from build123d import *

# Parameters (mm, degrees)
SKIZZE1_R                       = 48.5
AUFSATZ_LINEAR_AUSTRAGEN1_DEPTH = 5
SKIZZE2_W                       = 20
SKIZZE2_H                       = 13
AUFSATZ_LINEAR_AUSTRAGEN2_DEPTH = 20
SKIZZE3_W                       = 20
SKIZZE3_H                       = 2
AUFSATZ_LINEAR_AUSTRAGEN3_DEPTH = 23
SKIZZE4_R                       = 2.1
SCHNITT_LINEAR_AUSTRAGEN1_DEPTH = 74.003424577
FASE4_SIZE                      = 0.6
FASE6_SIZE                      = 2.5


with BuildPart() as part:
    # Skizze1 → Aufsatz-Linear austragen1 (new body)
    with BuildSketch(Plane(origin=(0, 0, 0), x_dir=(1, 0, 0), z_dir=(0, 1, 0))):
        with Locations(Location((0, 0, 0), (0, 0, 270))):
            Circle(SKIZZE1_R)
    extrude(amount=AUFSATZ_LINEAR_AUSTRAGEN1_DEPTH)

    # Skizze2 → Aufsatz-Linear austragen2 (add)
    with BuildSketch(Plane.XZ):
        with Locations((-27.5, 0)):
            Rectangle(SKIZZE2_W, SKIZZE2_H)
    extrude(amount=AUFSATZ_LINEAR_AUSTRAGEN2_DEPTH)

    # Skizze3 → Aufsatz-Linear austragen3 (add)
    with BuildSketch(Plane.XZ):
        with Locations((-27.5, 7.5)):
            Rectangle(SKIZZE3_W, SKIZZE3_H)
        with Locations((-27.5, -7.5)):
            Rectangle(SKIZZE3_W, SKIZZE3_H)
    extrude(amount=AUFSATZ_LINEAR_AUSTRAGEN3_DEPTH)

    # Skizze4 → Schnitt-Linear austragen1 (cut, through all)
    with BuildSketch(Plane.XZ.offset(20)):
        with Locations(Location((-32.5, 0, 0), (0, 0, 270))):
            Circle(SKIZZE4_R)
        with Locations(Location((-22.5, 0, 0), (0, 0, 270))):
            Circle(SKIZZE4_R)
    extrude(amount=-SCHNITT_LINEAR_AUSTRAGEN1_DEPTH, mode=Mode.SUBTRACT)

    # Fase4
    fase4_edges = [part.edges().sort_by_distance(p)[0] for p in [
        (0, 5, -48.5),
    ]]
    chamfer(fase4_edges, length=FASE4_SIZE)

    # Fase6
    fase6_edges = [part.edges().sort_by_distance(p)[0] for p in [
        (-32.5, 5, 2.1),
        (-22.5, 5, 2.1),
    ]]
    chamfer(fase6_edges, length=FASE6_SIZE)


solid = part.part
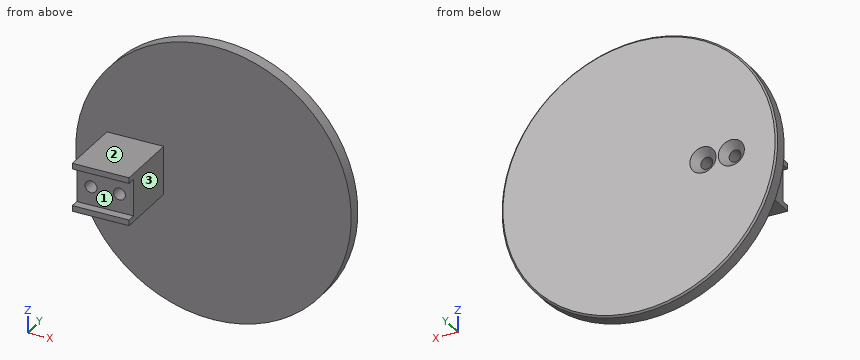
Geometry check sheet. Reference: the model listing, model coordinates, mm. Face numbers are marked on the shaded views. Give positions to 0.01 mm unless a question says otherwise; leave off trailing zeros. Write each loop counter-clockwise with the first axis right and the second up, starting at its lowest first coordinate (ties: lowest second). Pieces come first, ordered by that corner, then holes. Notation, with made-up numbers: M 81,86 L 97,86 A20 ccw 97,124 Z; hole C 22,55.5 d7. An arc over 180 degrees is marked long. One line per question, with ' | ' between items.
1. Cross-section at C-C (x = 0). Enter the section's corners in (y, z).
Ans:
outline: M 0,-48.5 L 4.4,-48.5 L 5,-47.9 L 5,47.9 L 4.4,48.5 L 0,48.5 Z
2. Cross-section at B-B (y = -12.75). Enter the section's corners in (x, z).
Ans:
outline: M -37.5,-8.5 L -17.5,-8.5 L -17.5,8.5 L -37.5,8.5 Z; hole C -32.5,0 d4.2; hole C -22.5,0 d4.2
3. Scan lines: line 1 along X through (y, z) = (-14.5, 0); line 2 along Y through (x, z) = (-24, -13); line 3 along X through (y, z) = (-1.5, 5.5). Record each from-to range of solid material in increasing order. Write a range as from..to.
Ans:
line 1: -37.5..-34.6, -30.4..-24.6, -20.4..-17.5 | line 2: 0..5 | line 3: -37.5..-17.5
4. Cross-section at A-A (z = 0). Enter the section's corners in (x, y).
Ans:
outline: M -48.5,0 L -37.5,0 L -37.5,-20 L -34.6,-20 L -34.6,2.5 L -37.1,5 L -47.9,5 L -48.5,4.4 Z; M -30.4,-20 L -24.6,-20 L -24.6,2.5 L -27.1,5 L -27.9,5 L -30.4,2.5 Z; M -20.4,-20 L -17.5,-20 L -17.5,0 L 48.5,0 L 48.5,4.4 L 47.9,5 L -17.9,5 L -20.4,2.5 Z
5. Mould release check, pull along Z, two halves, no side actions. Record for the marked faces 1, 2 and 3: released by +Z, released by -Z, zero draft, split by the parting line, or undercut.
Ans:
face 1: undercut | face 2: released by +Z | face 3: zero draft
6. Gauge pin test, flat ends, axial feed: pin 1 (6.5 mm diameter, centred on x = -22.5, z = 0, fed in from -Y); pin 2 (2 mm diameter, centred on y = -3.5, z = 7.5, fed in from -X); pin 3 (1.5 mm diameter, centred on y = -1, z = -21, fed in from -X); pin 4 (3.5 mm diameter, centred on x = -29, y = -22, fed in from +Z). Record the tip position at first contact, or that the pin passes through.
Ans:
pin 1: y = -20 | pin 2: x = -37.5 | pin 3: through | pin 4: z = 8.5
